Verification items for the finished model (mm, model axes). Coordinates: 2 decimals unless noted, no trailing zeros. Write each loop counter-clockwise with the first axis right and the second up, starting at its lowest first coordinate (ties: lowest second). Pieces come first, ordered by that corner, then holes. Notation, with made-up numbers: (79, 55) -> (129, 55) arc R33 ccw to (129, 89) -> close; hole circle Ø7 at (27.5, 16). An arc over 180 degrees is marked (long way). Use CSV: the item, a comma, the result in double quotes.
```python
from build123d import *

# Parameters (mm, degrees)
F0_W     = 11.8872
F0_H     = 2.881706
F0_H_2   = 2.588412
F2_R     = 2.7051
F3_DEPTH = 19.05


with BuildPart() as f1:
    # F0 (on Front) → F1 (revolve)
    with BuildSketch(Plane.XZ):
        with Locations((5.9436, 17.609147)):
            Rectangle(F0_W, F0_H)
        Polygon((11.8872, 16.168294), (0, 16.168294), (0.508, 15.875), (11.8872, 15.875), align=None)
        Polygon((0.508, 15.875), (0, 15.581706), (11.8872, 15.581706), (11.8872, 15.875), align=None)
        with Locations((5.9436, 14.2875)):
            Rectangle(F0_W, F0_H_2)
        Polygon((11.8872, 12.993294), (0, 12.993294), (0.508, 12.7), (11.8872, 12.7), align=None)
        Polygon((0.508, 12.7), (0, 12.406706), (11.8872, 12.406706), (11.8872, 12.7), align=None)
        with Locations((5.9436, 11.1125)):
            Rectangle(F0_W, F0_H_2)
        Polygon((11.8872, 9.818294), (0, 9.818294), (0.508, 9.525), (11.8872, 9.525), align=None)
        Polygon((0.508, 9.525), (0, 9.231706), (11.8872, 9.231706), (11.8872, 9.525), align=None)
        with Locations((5.9436, 7.9375)):
            Rectangle(F0_W, F0_H_2)
        Polygon((11.8872, 6.643294), (0, 6.643294), (0.508, 6.35), (11.8872, 6.35), align=None)
        Polygon((0.508, 6.35), (0, 6.056706), (11.8872, 6.056706), (11.8872, 6.35), align=None)
        with Locations((5.9436, 4.7625)):
            Rectangle(F0_W, F0_H_2)
        Polygon((11.8872, 3.468294), (0, 3.468294), (0.508, 3.175), (11.8872, 3.175), align=None)
        Polygon((0.508, 3.175), (0, 2.881706), (11.8872, 2.881706), (11.8872, 3.175), align=None)
        with Locations((5.9436, 1.5875)):
            Rectangle(F0_W, F0_H_2)
        Polygon((0, 0.293294), (0.508, 0), (11.8872, 0), (11.8872, 0.293294), align=None)
    revolve(axis=Axis((11.8872, 0, 9.525), (0, 0, -1)))

    # F2 (on face) → F3 (cut, through all)
    with BuildSketch(Plane.XY.offset(19.05)):
        with Locations((11.8872, 0)):
            Circle(F2_R)
    extrude(amount=-F3_DEPTH, mode=Mode.SUBTRACT)


solid = f1.part
```
1) Scan lines: L1, parallel to Y at x = 11.25, z = 14.5; L2, parallel to Y at x = 2.25, z = 18.25; L3, parallel to X at y = 8.5, z = 12.25. Record each from-to range of solid material in increasing order.
Return value:
L1,"-11.87 to -2.63, 2.63 to 11.87"
L2,"-6.96 to 6.96"
L3,"3.58 to 20.2"
2) Mould release check, pull along Z, two halves, no side actions. Record for faces 1 (the cylindrical face through (9.185, 0.119, 9.658)), 2 (the flat face through (9.5, -2.4, 0)), 3 (the conical face through (1, -4, 16)): released by +Z, released by -Z, zero draft, split by the parting line, or undercut.
Return value:
face 1,"zero draft"
face 2,"released by -Z"
face 3,"undercut"
3) Cross-section at A-A (z = 17.5). Record the boundary of the cut face in (x, y).
Return value:
outline,"circle Ø23.77 at (11.89, 0); hole circle Ø5.41 at (11.89, 0)"
4) Gauge pin test, flat ends, axial feed: pin 1 (8 mm diameter, centred on y = 5.5, z = 17, fed in from +X); pin 2 (6 mm diameter, centred on x = 8.5, z = 3.5, fed in from -Y); pin 3 (1 mm diameter, centred on x = 12, y = -1.5, fed in from -Z). Record the tip position at first contact, or that the pin passes through.
Return value:
pin 1,"x = 23.68"
pin 2,"y = -11.88"
pin 3,"through"
